```python
from build123d import *

# Parameters (mm, degrees)
SKIZZE1_R                       = 40
AUFSATZ_LINEAR_AUSTRAGEN1_DEPTH = 5
SKIZZE2_R                       = 10.75
SCHNITT_LINEAR_AUSTRAGEN1_DEPTH = 3
SKIZZE3_R                       = 3
SKIZZE3_R_2                     = 0.75
SCHNITT_LINEAR_AUSTRAGEN2_DEPTH = 13
SKIZZE4_W                       = 8
SKIZZE4_H                       = 8
AUFSATZ_LINEAR_AUSTRAGEN2_DEPTH = 18.97
AUFSATZ_LINEAR_AUSTRAGEN3_DEPTH = 8
AUFSATZ_LINEAR_AUSTRAGEN4_DEPTH = 8
SKIZZE7_R                       = 1.75
SCHNITT_LINEAR_AUSTRAGEN3_DEPTH = 33.27
SKIZZE9_W                       = 40.738044429
SKIZZE9_H                       = 4
AUFSATZ_LINEAR_AUSTRAGEN5_DEPTH = 20
SKIZZE10_R                      = 3
AUFSATZ_LINEAR_AUSTRAGEN6_DEPTH = 4
SKIZZE11_W                      = 0.727428481
SKIZZE11_H                      = 19.15
SKIZZE11_W_2                    = 0.206337284
SCHNITT_LINEAR_AUSTRAGEN4_DEPTH = 16.39


with BuildPart() as part:
    # Skizze1 → Aufsatz-Linear austragen1 (new body)
    with BuildSketch(Plane(origin=(0, 0, 0), x_dir=(1, 0, 0), z_dir=(0, 1, 0))):
        with Locations(Location((0, 0, 0), (0, 0, 270))):
            Circle(SKIZZE1_R)
    extrude(amount=AUFSATZ_LINEAR_AUSTRAGEN1_DEPTH)

    # Skizze2 → Schnitt-Linear austragen1 (cut)
    with BuildSketch(Plane.XZ):
        with Locations(Location((0, 0, 0), (0, 0, 270))):
            Circle(SKIZZE2_R)
    extrude(amount=-SCHNITT_LINEAR_AUSTRAGEN1_DEPTH, mode=Mode.SUBTRACT)

    # Skizze3 → Schnitt-Linear austragen2 (cut)
    with BuildSketch(Plane.XZ):
        with Locations(Location((0, 0, 0), (0, 0, 270))):
            Circle(SKIZZE3_R)
        with Locations(Location((-0.185951444, 7.49769445, 0), (0, 0, 270))):
            Circle(SKIZZE3_R_2)
        with Locations(Location((7.49769445, 0.185951444, 0), (0, 0, 270))):
            Circle(SKIZZE3_R_2)
        with Locations(Location((0.185951444, -7.49769445, 0), (0, 0, 270))):
            Circle(SKIZZE3_R_2)
        with Locations(Location((-7.49769445, -0.185951444, 0), (0, 0, 270))):
            Circle(SKIZZE3_R_2)
    extrude(amount=-SCHNITT_LINEAR_AUSTRAGEN2_DEPTH, mode=Mode.SUBTRACT)

    # Skizze4 → Aufsatz-Linear austragen2 (add)
    with BuildSketch(Plane(origin=(0, 5, 0), x_dir=(1, 0, 0), z_dir=(0, 1, 0))):
        with Locations((-13.649547585, -4.604184577)):
            Rectangle(SKIZZE4_W, SKIZZE4_H)
        with Locations((35.098787181, -4.555000776)):
            Rectangle(SKIZZE4_W, SKIZZE4_H)
    extrude(amount=AUFSATZ_LINEAR_AUSTRAGEN2_DEPTH)

    # Skizze5 → Aufsatz-Linear austragen3 (add)
    with BuildSketch(Plane(origin=(39.098787181, 0, 0), x_dir=(0, 0, -1), z_dir=(1, 0, 0))):
        Polygon((-0.555000776, 23.97), (7.911534589, 5), (-0.555000776, 5), align=None)
    extrude(amount=-AUFSATZ_LINEAR_AUSTRAGEN3_DEPTH)

    # Skizze6 → Aufsatz-Linear austragen4 (add)
    with BuildSketch(Plane.ZY.offset(17.649547585)):
        Polygon((0.604184577, 23.97), (-7.911534589, 5), (0.604184577, 5), align=None)
    extrude(amount=-AUFSATZ_LINEAR_AUSTRAGEN4_DEPTH)

    # Skizze7 → Schnitt-Linear austragen3 (cut)
    with BuildSketch(Plane.XY.offset(8.604184577)):
        with Locations((-13.944175516, 20)):
            Circle(SKIZZE7_R)
        with Locations((-13.944175516, 10)):
            Circle(SKIZZE7_R)
        with Locations(Location((34.90415925, 10, 0), (0, 0, 90))):
            Circle(SKIZZE7_R)
        with Locations(Location((34.908787181, 20, 0), (0, 0, 90))):
            Circle(SKIZZE7_R)
    extrude(amount=-SCHNITT_LINEAR_AUSTRAGEN3_DEPTH, mode=Mode.SUBTRACT)

    # Skizze9 → Aufsatz-Linear austragen5 (add)
    with BuildSketch(Plane(origin=(0, 5, 0), x_dir=(1, 0, 0), z_dir=(0, 1, 0))):
        with Locations((10.767809396, 20.99827279)):
            Rectangle(SKIZZE9_W, SKIZZE9_H)
    extrude(amount=AUFSATZ_LINEAR_AUSTRAGEN5_DEPTH)

    # Skizze10 → Aufsatz-Linear austragen6 (add)
    with BuildSketch(Plane(origin=(0, 0, -22.99827279), x_dir=(-1, 0, 0), z_dir=(0, 0, -1))):
        with Locations(Location((0.044175516, 15, 0), (0, 0, 180))):
            Circle(SKIZZE10_R)
    extrude(amount=AUFSATZ_LINEAR_AUSTRAGEN6_DEPTH)

    # Skizze11 → Schnitt-Linear austragen4 (cut)
    with BuildSketch(Plane.XY.offset(8.604184577)):
        with Locations((-9.96492706, 14.575)):
            Rectangle(SKIZZE11_W, SKIZZE11_H)
        with Locations((31.201955823, 14.575)):
            Rectangle(SKIZZE11_W_2, SKIZZE11_H)
    extrude(amount=-SCHNITT_LINEAR_AUSTRAGEN4_DEPTH, mode=Mode.SUBTRACT)


solid = part.part
```
For this review, take the finished solid that the model builds, in its own axes (mm). A direction names the side the tool comes from. Coordinates: 2 decimals unless noted, no trailing zeros. Loops run counter-clockwise (first coordinate to the right, second up) from the corner with the lowest first, then second, coordinate; pieces in that order, holes last. Notation, with made-up numbers: (22, 77) -> (50, 77) arc R20 cw to (50, 87) -> close; hole circle Ø2 at (63, 87.25). An arc over 180 degrees is marked (long way). Return JSON: item names as keys, results as strings. Group by question number.
(1) Tool access review of faces 5 (the flat face through (39.099, 15, 2)), 6 (the flat face through (-2.24, 3, -2.24)): name each direction out of +Z, -Z, +X, -X, +Y, -Y from which nothing blocks a thin tool from reaching the whole face with its end or side.
(2) Consider section D-D, the plane x = -22.5. Give the boundary of the cut face in (y, z), plus the area to 3 significant figures.
(3) Consider section C-C, the plane y = 15. Give the boundary of the cut face in (x, z) (3 decimals).
(4) Mouldability with a two-part tool opening along Y and no side actions: class faces 1 (the cylindrical face through (-0.69, 17.93, -24.97)), 2 (the cylindrical face through (-13.137, 18.447, 3.394)), 3 (the flat face through (-17.65, 15, 2)), 4 (the flat face through (-8, 0, 8)) as pulls with the +Y half, pulls with the -Y half, needs draft (parallel to the pull), parting line crosses it, or undercut.
(5) For pin 1 Ø8 at (y, z) = (18, 1.5) entering from +X; pin 2 Ø13 at (y, z) = (11, -1.5) entering from -X; pin 3 Ø1.5 at (x, z) = (23, 26.5) entering from +Y; pin 4 Ø12 at (x, z) = (-24, -29.5) entering from -Y, all flat-tipped, find the tip position at first contact; note any pin that passes through.
(6) To check wall thickness, follow L1, parallel to Y at x = -32, z = -20; L2, parallel to Z at x = 12, y = 9.5; L3, parallel to Z at x = 2, y = 16.25. State the ranges of each line that lie inside material, in increasing order.
(7) Consider section A-A, the plane y = 10. Give the boundary of the cut face in (x, z) (3 decimals), plus the area to 3 significant figures.
(8) Consider section B-B, the plane y = 1.75. Give the boundary of the cut face in (x, z), plus the area to 3 significant figures.
Results below:
{
 "1": {"face 5": "+Z, -Z, +X, +Y", "face 6": "-Y"},
 "2": {"outline": "(0, -33.07) -> (5, -33.07) -> (5, 33.07) -> (0, 33.07) -> close", "area": "331 mm2"},
 "3": {"outline": "(-17.65, -3.422) -> (-10.329, -3.422) -> (-10.329, 8.604) -> (-17.65, 8.604) -> close; (-9.601, -22.998) -> (-3.044, -22.998) -> (-3.044, -26.998) -> (2.956, -26.998) -> (2.956, -22.998) -> (31.137, -22.998) -> (31.137, -18.998) -> (-9.601, -18.998) -> close; (31.305, -3.448) -> (39.099, -3.448) -> (39.099, 8.555) -> (31.305, 8.555) -> close"},
 "4": {"face 1": "undercut", "face 2": "undercut", "face 3": "needs draft", "face 4": "pulls with the -Y half"},
 "5": {"pin 1": "stops at x = 39.1", "pin 2": "stops at x = -40", "pin 3": "stops at y = 5", "pin 4": "stops at y = 0"},
 "6": {"L1": "y = 0 to 5", "L2": "z = -23 to -19", "L3": "z = -27 to -19"},
 "7": {"outline": "(-17.65, -5.667) -> (-15.694, -5.667) -> (-15.694, 8.604) -> (-17.65, 8.604) -> close; (-12.194, -5.667) -> (-10.329, -5.667) -> (-10.329, 8.604) -> (-12.194, 8.604) -> close; (-9.601, -22.998) -> (31.137, -22.998) -> (31.137, -18.998) -> (-9.601, -18.998) -> close; (31.305, -5.68) -> (33.154, -5.68) -> (33.154, 8.555) -> (31.305, 8.555) -> close; (36.654, -5.68) -> (39.099, -5.68) -> (39.099, 8.555) -> (36.654, 8.555) -> close", "area": "279 mm2"},
 "8": {"outline": "circle Ø80 at (0, 0); hole circle Ø21.5 at (0, 0)", "area": "4,660 mm2"}
}
